Here's how the part is built. I have some questions about the finished solid (model axes, mm). Face numbers are marked on the shaded views. A direction names the side the tool comes from. Give positions to 0.01 mm unless a question says otherwise; leave off trailing zeros. Write each loop counter-clockwise with the first axis right and the second up, starting at its lowest first coordinate (ties: lowest second). Pieces come first, ordered by that corner, then holes. Notation, with made-up numbers: (85, 64) -> (117, 64) arc R20 ccw to (117, 100) -> close; hole circle Ø7 at (30, 32). An arc over 180 degrees is marked (long way). Answer as CSV lines item,"result". Start each with the question number.
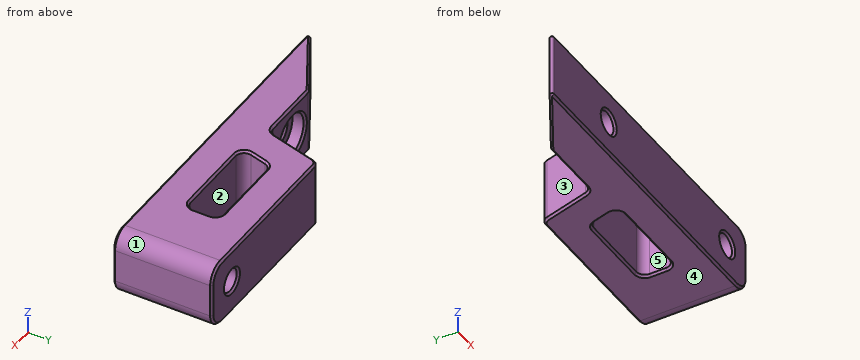
from build123d import *

# Parameters (mm, degrees)
BOSS_EXTRUDE1_DEPTH     = 6.35
CUT_EXTRUDE1_DEPTH      = 38.567106623
CUT_EXTRUDE1_DEPTH_BACK = 38.567106623
SKETCH2_R               = 2.1828125
SKETCH3_R               = 4.191
CUT_EXTRUDE2_DEPTH      = 2.54
FILLET1_R               = 0.396875
FILLET2_R               = 1.5875
FILLET3_R               = 3.175
CHAMFER1_SIZE           = 0.396875


with BuildPart() as part:
    # Sketch1 → Boss-Extrude1 (new, symmetric)
    with BuildSketch(Plane.XY):
        Polygon((-31.75, 0), (31.75, 0), (31.75, 19.05), (-2.324261314, 19.05), (-5.301846715, 7.9375), (-18.001846715, 7.9375), align=None)
        Polygon((19.05, 12.7), (19.05, 6.35), (0.846787688, 6.35), (2.54826506, 12.7), align=None, mode=Mode.SUBTRACT)
    extrude(amount=BOSS_EXTRUDE1_DEPTH, both=True)

    # Sketch2 → Cut-Extrude1 (cut, two sides: drawn at the far end of the back side and taken through both)
    with BuildSketch(Plane.XZ.offset(-CUT_EXTRUDE1_DEPTH_BACK)):
        with Locations(Location((-12.7, 0, 0), (0, 0, 270))):
            Circle(SKETCH2_R)
        with Locations(Location((25.4, 0, 0), (0, 0, 270))):
            Circle(SKETCH2_R)
    extrude(amount=CUT_EXTRUDE1_DEPTH + CUT_EXTRUDE1_DEPTH_BACK, mode=Mode.SUBTRACT)

    # Sketch3 → Cut-Extrude2 (cut)
    with BuildSketch(Plane(origin=(0, 7.9375, 0), x_dir=(1, 0, 0), z_dir=(0, 1, 0))):
        with Locations(Location((-12.7, 0, 0), (0, 0, 180))):
            Circle(SKETCH3_R)
    extrude(amount=-CUT_EXTRUDE2_DEPTH, mode=Mode.SUBTRACT)

    # Fillet1
    fillet1_edges = [part.edges().sort_by_distance(p)[0] for p in [
        (-31.75, 0, 0),
    ]]
    fillet(fillet1_edges, radius=FILLET1_R)

    # Fillet2
    fillet2_edges = [part.edges().sort_by_distance(p)[0] for p in [
        (-18.001846715, 7.9375, 0),
        (-5.301846715, 7.9375, 0),
        (-2.324261314, 19.05, 0),
        (19.05, 12.7, 0),
        (2.54826506, 12.7, 0),
        (0.846787688, 6.35, 0),
        (19.05, 6.35, 0),
    ]]
    fillet(fillet2_edges, radius=FILLET2_R)

    # Fillet3
    fillet3_edges = [part.edges().sort_by_distance(p)[0] for p in [
        (31.75, 9.525, 6.35),
        (31.75, 9.525, -6.35),
    ]]
    fillet(fillet3_edges, radius=FILLET3_R)

    # Chamfer1
    chamfer1_edges = [part.edges().sort_by_distance(p)[0] for p in [
        (31.75, 19.05, 0),
        (31.75, 0, 0),
        (13.73443514, 19.05, -6.35),
        (13.73443514, 19.05, 6.35),
        (30.82006403, 19.05, 5.42006403),
        (30.82006403, 19.05, -5.42006403),
        (30.82006403, 0, 5.42006403),
        (30.82006403, 0, -5.42006403),
        (-12.7, 0, 2.1828125),
        (25.4, 19.05, 2.1828125),
        (25.4, 0, 2.1828125),
        (-8.509, 7.9375, 0),
        (-12.7, 5.3975, 2.1828125),
        (-0.846921168, 0, -6.35),
        (-0.846921168, 0, 6.35),
        (-30.652194148, 0.294156191, -6.35),
        (-30.652194148, 0.294156191, 6.35),
        (-12.04822784, 7.9375, -6.35),
        (-12.04822784, 7.9375, 6.35),
        (-3.813054014, 13.49375, -6.35),
        (-3.813054014, 13.49375, 6.35),
        (-24.418753604, 4.23269708, -6.35),
        (-24.418753604, 4.23269708, 6.35),
        (19.05, 9.525, -6.35),
        (10.614448327, 12.7, -6.35),
        (1.807620061, 9.935875234, -6.35),
        (10.189078984, 6.35, -6.35),
        (-2.072538489, 18.721948428, -6.35),
        (-17.987352606, 7.883407249, -6.35),
        (10.614448327, 12.7, 6.35),
        (19.05, 9.525, 6.35),
        (10.189078984, 6.35, 6.35),
        (1.807620061, 9.935875234, 6.35),
        (-2.072538489, 18.721948428, 6.35),
        (-17.987352606, 7.883407249, 6.35),
        (-5.55356954, 8.265551572, -6.35),
        (-5.55356954, 8.265551572, 6.35),
        (1.656209539, 6.971091231, -6.35),
        (1.656209539, 6.971091231, 6.35),
        (2.799987885, 12.371948428, -6.35),
        (2.799987885, 12.371948428, 6.35),
        (18.585032015, 12.235032015, -6.35),
        (18.585032015, 12.235032015, 6.35),
        (18.585032015, 6.814967985, -6.35),
        (18.585032015, 6.814967985, 6.35),
    ]]
    chamfer(chamfer1_edges, length=CHAMFER1_SIZE - 0.0001)  # a hair under: the kernel refuses the full size


solid = part.part
Item 1: We'd pull the mould along Y, two halves only. Please class the marked faces 3, 4 and 5: released by +Y, released by -Y, zero draft, split by the parting line, or undercut.
Item 2: If I drill on line 1 (Z direction, x = 25.4, y = 14); line 2 (Y direction, x = 8, z = -1.5); line 3 (Z direction, x = -12.7, y = 6.1), over which ranges is the centre line in solid material (lowest first)? Write a range as [from, to].
Item 3: If we section it at C-C (z = 0): State how many separate pieces and enclosed holes the cut face has, and give its area (3 significant figures).
Item 4: If we section it at D-D (x = 14): Please give me the cut outline in (y, z), and give its area (3 significant figures).
Item 5: If we section it at B-B (y = 14.5): Please give me the cut outline in (x, z) (3 decimals), and give its area (3 significant figures).
Item 6: For the marked faces 1 and 2, which set-ups out of +Z, -Z, +X, -X, +Y, -Y let a thin tool reach every point of the face, with its end or its side?
Item 7: If we section it at A-A (x = -12.7): Please give me the cut outline in (y, z), and give its area (3 significant figures).
Item 8: I'm going to push flat-ended pins straight in: pin 1 (1 mm diameter, centred on x = 24.5, z = 0, fed in from -Y); pin 2 (5.5 mm diameter, centred on x = -12.5, z = 1, fed in from +Y); pin 3 (5 mm diameter, centred on x = -12.7, z = 0, fed in from -Y); pin 4 (5 mm diameter, centred on y = 13.5, z = -4.5, fed in from -X). Where does each tip first touch, or does it pass through?
Final values:
1,face 3,"released by +Y"
1,face 4,"zero draft"
1,face 5,"undercut"
2,line 1,"[-6.35, -2.18], [2.18, 6.35]"
2,line 2,"[0, 6.35], [12.7, 19.05]"
2,line 3,"[-6.35, -4.19], [4.19, 6.35]"
3,separate pieces,"3"
3,enclosed holes,"1"
3,area,"607 mm2"
4,outline,"(0, -5.95) -> (0.4, -6.35) -> (5.95, -6.35) -> (6.35, -5.95) -> (6.35, 5.95) -> (5.95, 6.35) -> (0.4, 6.35) -> (0, 5.95) -> close; (12.7, -5.95) -> (13.1, -6.35) -> (18.65, -6.35) -> (19.05, -5.95) -> (19.05, 5.95) -> (18.65, 6.35) -> (13.1, 6.35) -> (12.7, 5.95) -> close"
4,area,"161 mm2"
5,outline,"(-3.543, -5.953) -> (-3.133, -6.35) -> (28.575, -6.35) arc R3.175 ccw to (31.75, -3.175) -> (31.75, 3.175) arc R3.175 ccw to (28.575, 6.35) -> (-3.133, 6.35) -> (-3.543, 5.953) -> close; hole circle Ø4.366 at (25.4, 0)"
5,area,"429 mm2"
6,face 1,"+Z, +X, +Y, -Y"
6,face 2,"+Z, -Z"
7,outline,"(0, -5.95) -> (0.4, -6.35) -> (7.54, -6.35) -> (7.94, -5.95) -> (7.94, -4.59) -> (7.54, -4.19) -> (5.4, -4.19) -> (5.4, -2.58) -> (5, -2.18) -> (0.4, -2.18) -> (0, -2.58) -> close; (0, 2.58) -> (0.4, 2.18) -> (5, 2.18) -> (5.4, 2.58) -> (5.4, 4.19) -> (7.54, 4.19) -> (7.94, 4.59) -> (7.94, 5.95) -> (7.54, 6.35) -> (0.4, 6.35) -> (0, 5.95) -> close"
7,area,"55.2 mm2"
8,pin 1,"through"
8,pin 2,"y = 5.4"
8,pin 3,"y = 0.08"
8,pin 4,"x = -4.48"
